Input: dimensioned drawing with shaded views. Units: mm. Origin: part minimum x, y, z. Coordinates: 2 decimals unless noted, no trailing zeros. Order: outer loops, then holes, each group sorted by start corner. A loop starts at its lowest first (then second) coordinate and runs counter-clockwise, first axis right, second up. Notation, with made-up numbers: M 41,57.25 L 73,57.25 A25 ccw 73,95.25 Z; hole C -39.75,-14.5 d3. An arc over 180 degrees is marked long. Write item = value, one per line.
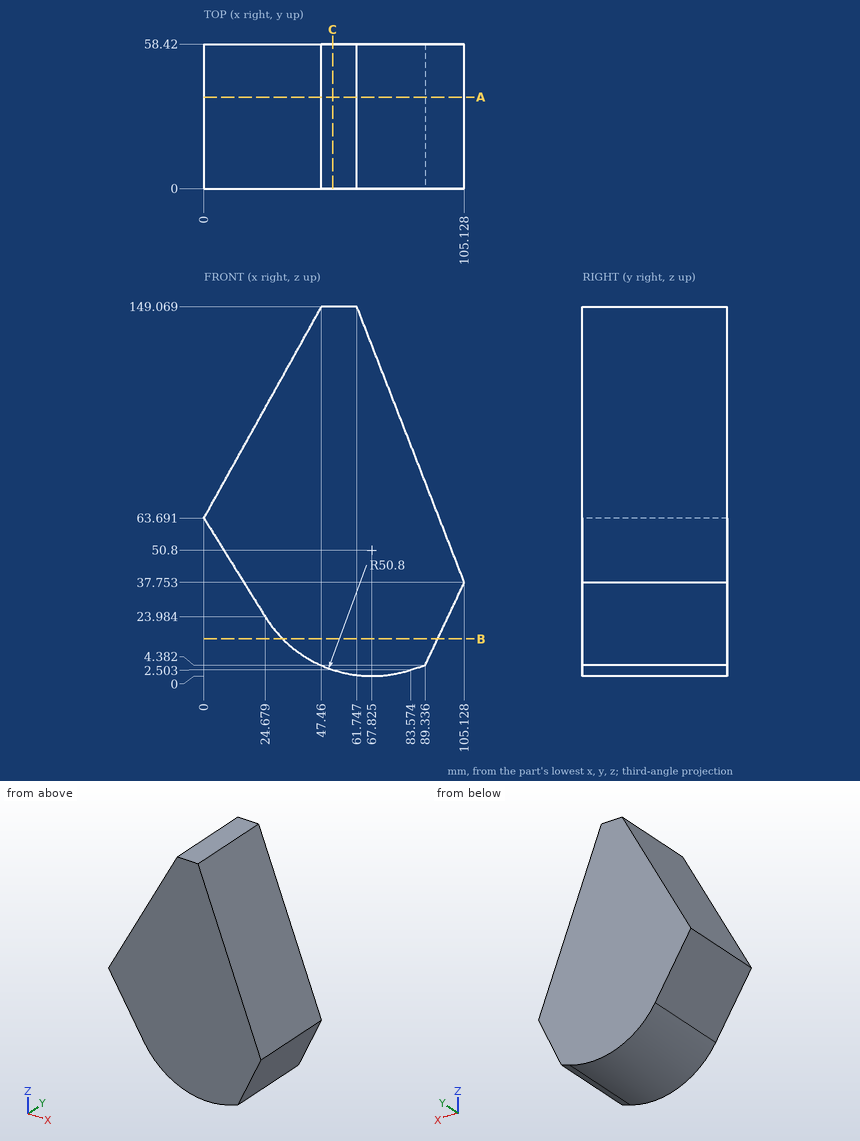
1) Section A-A, the plane y = 37. Return loops of the section in (x, z) (1 decimal).
Numbers:
outline = M 0,63.7 L 24.7,24 A50.8 ccw 83.6,2.5 L 89.3,4.4 L 105.1,37.8 L 61.7,149.1 L 47.5,149.1 Z
2) Section B-B, the plane z = 15. Return loops of the section in (x, y).
Numbers:
outline = M 31.78,0 L 94.36,0 L 94.36,58.42 L 31.78,58.42 Z
3) Section C-C, the plane x = 52. Return loops of the section in (y, z).
Numbers:
outline = M 0,2.53 L 58.42,2.53 L 58.42,149.07 L 0,149.07 Z
4) Pin query (flat end, axial travel): pin 1 (12 mm diameter, centred on x = 78, z = 133.5, fed in from -Y); pin 2 (10 mm diameter, centred on y = 9, z = 88, fed in from +X) (1 decimal); pin 3 (2 mm diameter, centred on y = 40.5, z = 102, fed in from +X); pin 4 (10 mm diameter, centred on y = 15, z = 94.5, fed in from +X). Return the tip coordinate at first contact, or that it passes through.
Numbers:
pin_1 = through
pin_2 = 87.5
pin_3 = 80.48
pin_4 = 84.96
5) Line query: L1, parallel to Z at x = 19, y = 56.5 (1 decimal); L2, parallel to X at y = 20.5, z = 119.5 (1 decimal); L3, parallel to X at y = 5, z = 124 (1 decimal). Output: solid intervals per line, ascending.
Numbers:
L1 = 33.1 to 97.9
L2 = 31 to 73.3
L3 = 33.5 to 71.5
